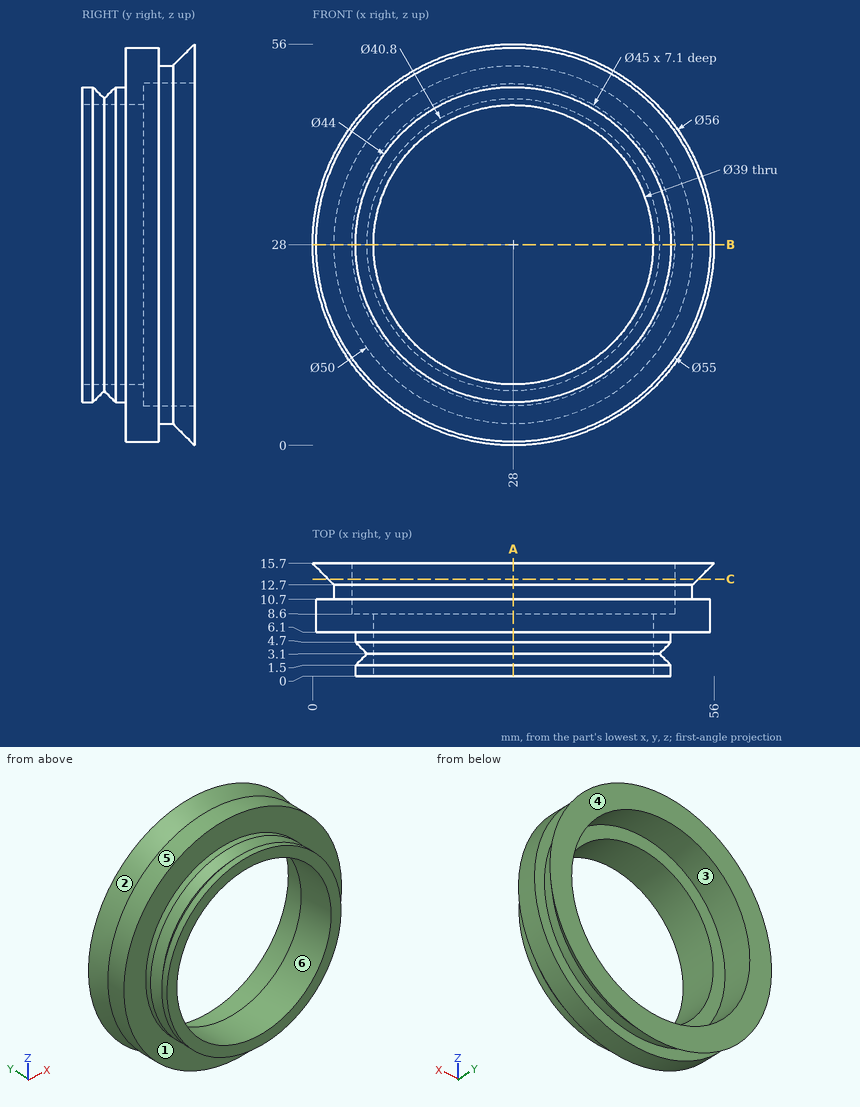
Check sheet for the drawn part. Datum: minimum x, y, z corner. Units: mm. A direction names the side the tool comes from. Coordinates: 2 decimals unless noted, no trailing zeros. Order: outer loops, then holes, each group sorted by start corner. A loop starts at its lowest first (then second) coordinate and runs counter-clockwise, first axis right, second up. Notation, with made-up numbers: M -1,34 L 47,34 A21 ccw 47,65 Z; hole C -30,31 d5. An arc over 180 degrees is marked long. One line per item, written item: value. Start each with the question number.
Item 1: Access from +Z, -Z, +X, -X, +Y, -Y to the whole of each face (thin tool, end or side, straight path). Record for the marked faces 1, 2 and 3.
Item 2: Mould release check, pull along Z, two halves, no side actions. Record for the marked faces 4, 5 and 6: released by +Z, released by -Z, zero draft, split by the parting line, or undercut.
Item 3: Scan lines: probe 1 along Z at (x, y) = (28, 12.5); probe 2 along Z at (x, y) = (28, 5). Record each from-to range of solid material in increasing order.
Item 4: Sectioned sample at C-C (y = 13.5). Enter the section's corners in (x, z).
Item 5: Gauge pin test, flat ends, axial feed: pin 1 (6 mm diameter, centred on y = 4.5, z = 9.5, fed in from +X); pin 2 (13.5 mm diameter, centred on x = 25.5, z = 19, fed in from +Y); pin 3 (1 mm diameter, centred on x = 34.5, y = 3, fed in from -Z); pin 4 (1.5 mm diameter, centred on x = 42.5, z = 46.5, fed in from -Y). Record the tip position at first contact, or that the pin passes through.
Item 6: Sectioned sample at B-B (z = 28). Enter the section's corners in (x, y).
Item 7: Sectioned sample at A-A (x = 28). Enter the section's corners in (y, z), then the cut area to 3 significant figures.
Conclusion:
1. face 1: -Y
1. face 2: none
1. face 3: +Y
2. face 4: zero draft
2. face 5: split by the parting line
2. face 6: undercut
3. probe 1: z = 3 to 5.5, 50.5 to 53
3. probe 2: z = 6 to 8.5, 47.5 to 50
4. outline: C 28,28 d51.6; hole C 28,28 d45
5. pin 1: stops at x = 50.39
5. pin 2: passes through
5. pin 3: stops at z = 8.01
5. pin 4: stops at y = 6.1
6. outline: M 0,15.7 L 3,12.7 L 3,10.7 L 0.5,10.7 L 0.5,6.1 L 6,6.1 L 6,4.7 L 7.6,3.1 L 6,1.5 L 6,0 L 8.5,0 L 8.5,8.6 L 5.5,8.6 L 5.5,15.7 Z; M 47.5,0 L 50,0 L 50,1.5 L 48.4,3.1 L 50,4.7 L 50,6.1 L 55.5,6.1 L 55.5,10.7 L 53,10.7 L 53,12.7 L 56,15.7 L 50.5,15.7 L 50.5,8.6 L 47.5,8.6 Z
7. outline: M 0,6 L 1.5,6 L 3.1,7.6 L 4.7,6 L 6.1,6 L 6.1,0.5 L 10.7,0.5 L 10.7,3 L 12.7,3 L 15.7,0 L 15.7,5.5 L 8.6,5.5 L 8.6,8.5 L 0,8.5 Z; M 0,47.5 L 8.6,47.5 L 8.6,50.5 L 15.7,50.5 L 15.7,56 L 12.7,53 L 10.7,53 L 10.7,55.5 L 6.1,55.5 L 6.1,50 L 4.7,50 L 3.1,48.4 L 1.5,50 L 0,50 Z
7. area: 120 mm^2
